Input: part model. Units: mm. Frame: model coordinates. Coordinates: 2 decimals unless noted, no trailing zeros. Loops run counter-clockwise (first coordinate to the right, second up) from the corner with the lowest first, then second, coordinate; pieces in that order, holes last. Notation, with made-up numbers: (75, 18) -> (118, 18) arc R16 ccw to (118, 42) -> close; hole circle Ø8 at (42, 9.25). An arc over 180 degrees is marked (long way). Put each result on its own line as item: value. Start each with the question number.
1) Material intervals for L1, parallel to X at y = 4.5, z = 0; L2, parallel to Z at x = -2, y = 6.75; L3, parallel to Z at x = 0.5, y = 6, sorted ascending.
2) Cut plane A-A (x = 0). Return the cut outline in (y, z), plus the area to 3 significant figures.
3) Contact query for a flat-ended pin moving along its axis: P1, Ø7.5, axis at x = 0, z = 0, coming from the +Y side. Output: stop coordinate, or through.
4) Pull-direction query (X, two-part tool) for faces 1 (the flat face through (-11.759, 5, 1)), 2 (the flat face through (0, 5, 3.8)), 3 (the cylindrical face through (0.165, 4.93, -4.697)), 4 (the flat face through (1, 5, 8.642)); classes: pulls with the +X half, pulls with the -X half, needs draft (parallel to the pull), parting line crosses it, or undercut.
5) Cut plane B-B (y = 0.5). Return the cut outline in (x, z), plus the area to 3 significant figures.
6) Cut plane C-C (z = 0). Return the cut outline in (x, y), plus the area to 3 significant figures.
from build123d import *

# Parameters (mm, degrees)
SKETCH1_W           = 25.499374977
SKETCH1_H           = 15.79332804
BOSS_EXTRUDE1_DEPTH = 10


with BuildPart() as part:
    # Sketch1 → Boss-Extrude1 (new body)
    with BuildSketch(Plane(origin=(0, 0, 0), x_dir=(1, 0, 0), z_dir=(0, 1, 0))):
        with Locations((0.990737135, -0.745657883)):
            Rectangle(SKETCH1_W, SKETCH1_H)
        with BuildLine():
            Line((-2.765863337, -3.8), (2.765863337, -3.8))
            ThreePointArc((2.765863337, -3.8), (0, 4.7), (-2.765863337, -3.8))
        make_face(mode=Mode.SUBTRACT)
    extrude(amount=BOSS_EXTRUDE1_DEPTH)


solid = part.part
Results found:
1. L1: x = -11.76 to -4.7, 4.7 to 13.74
1. L2: z = -7.15 to -4.25, 3.8 to 8.64
1. L3: z = -7.15 to -4.67, 3.8 to 8.64
2. outline: (0, -7.15) -> (10, -7.15) -> (10, -4.7) -> (0, -4.7) -> close; (0, 3.8) -> (10, 3.8) -> (10, 8.64) -> (0, 8.64) -> close
2. area: 72.9 mm2
3. P1: passes through
4. face 1: pulls with the -X half
4. face 2: undercut
4. face 3: undercut
4. face 4: needs draft
5. outline: (-11.76, -7.15) -> (13.74, -7.15) -> (13.74, 8.64) -> (-11.76, 8.64) -> close; hole (-2.77, 3.8) arc R4.7 ccw (long way) to (2.77, 3.8) -> close
5. area: 337 mm2
6. outline: (-11.76, 0) -> (-4.7, 0) -> (-4.7, 10) -> (-11.76, 10) -> close; (4.7, 0) -> (13.74, 0) -> (13.74, 10) -> (4.7, 10) -> close
6. area: 161 mm2
